Autodesk Inventor part; units mm, degrees
ref_plane "YZ Plane" through (0, 0, 0) normal (1, 0, 0) x (0, 1, 0)
ref_plane "XZ Plane" through (0, 0, 0) normal (0, 1, 0) x (-1, 0, 0)
ref_plane "XY Plane" through (0, 0, 0) normal (0, 0, 1) x (1, 0, 0)
sketch "Sketch1" plane through (0, 0, 0) normal (0, 0, 1) x (1, 0, 0)
  line L0 (0, 0) -> (190.5, 0)
  line L1 (190.5, 0) -> (190.5, 254)
  line L2 (190.5, 254) -> (0, 254)
  line L3 (0, 254) -> (0, 0)
  dimension "d0" = 190.5
  dimension "d1" = 254
extrude "Extrusion1" add sketch "Sketch1" against normal blind 25.4
sketch "Sketch2" plane through (0, 0, 0) normal (0, 0, 1) x (1, 0, 0)
  line L0 (0, 0) -> (0, 254)
  line L1 (0, 127) -> (190.5, 127)
  line L2 (190.5, 254) -> (190.5, 0)
  line L3 (54.1274, 112.395) -> (54.1274, 106.045)
  line L4 (95.25, 144.145) -> (117.3226, 144.145)
  line L5 (117.3226, 144.145) -> (73.1774, 144.145)
  line L6 (95.25, 109.855) -> (117.3226, 109.855)
  line L7 (117.3226, 109.855) -> (73.1774, 109.855)
  line L8 (73.1774, 144.145) -> (117.3226, 144.145)
  line L9 (117.3226, 144.145) -> (117.3226, 150.495)
  line L10 (117.3226, 150.495) -> (73.1774, 150.495)
  line L11 (73.1774, 150.495) -> (73.1774, 144.145)
  line L12 (73.1774, 109.855) -> (117.3226, 109.855)
  line L13 (117.3226, 109.855) -> (117.3226, 103.505)
  line L14 (117.3226, 103.505) -> (73.1774, 103.505)
  line L15 (73.1774, 103.505) -> (73.1774, 109.855)
  point P0 (54.1274, 141.605)
  dimension "d16" = 22.0726
  dimension "d17" = 44.1452
  dimension "d18" = 6.35
  dimension "d19" = 6.35
extrude "Extrusion2" add sketch "Sketch2" along normal blind 76.2
sketch "Sketch3" plane through (54.1274, 112.395, 0) normal (0, 1, 0) x (1, 0, 0)
  circle A0 centre (22.0726, -63.5) radius 6.35
  point P0 (-54.1274, 0)
  dimension "d10" = 12.7
extrude "Extrusion3" [suppressed]
sketch "Sketch4" plane through (0, 0, -25.4) normal (0, 0, -1) x (-1, 0, 0)
  line L0 (-190.5, 0) -> (-190.5, 254)
  line L1 (0, 0) -> (-190.5, 0)
  line L2 (-190.5, 0) -> (-190.5, 12.7)
  line L3 (-190.5, 12.7) -> (0, 12.7)
  line L4 (0, 12.7) -> (0, 0)
  dimension "d13" = 12.7
extrude "Extrusion4" add sketch "Sketch4" along normal blind 228.6
sketch "Sketch5" plane through (73.1774, 150.495, 0) normal (0, 1, 0) x (1, 0, 0)
  circle A0 centre (22.0726, -63.5) radius 6.35
  point P0 (-73.1774, 0)
  dimension "d20" = 12.7
extrude "Extrusion5" cut sketch "Sketch5" against normal blind 101.6
properties part number "LucasCharles Part3" material "ABS Plastic"
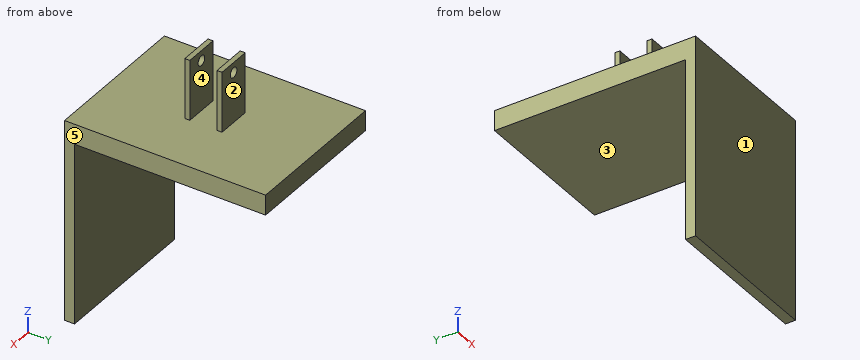
Design review of the part built by this model. Coordinates are the model's own, in mm. Face numbers are marked on the shaded views. A direction names the side the tool comes from. Round coordinates to 2 decimals unless told otherwise and drop trailing zeros. Write each loop counter-clockwise with the first axis right and the second up, starting at its lowest first coordinate (ties: lowest second). Pieces come first, ordered by that corner, then holes. Notation, with made-up numbers: (73.5, -25) - (85.5, -25) arc R38 cw to (85.5, 13) - close; hole circle Ø6 at (4.5, 61). An arc over 180 degrees is marked (long way). Use a Markdown table: item, result. Add a question column.
1. We need section B-B (z = 63.5). State the section outline as (x, y) points (3 decimals).
2. Wall thickness on probe 1 along X at (y, z) = (148, 63); probe 2 along Z at (x, y) = (95.25, 148); probe 3 along Y at (x, z) = (88, 32) (3 decimals): over which ranges is each line inside the solid? List them lowest first.
3. For the marked faces 1, 2, 3, 4 and 5, list the 3-axis set-ups (+Z, -Z, +X, -X, +Y, -Y) from which the entire face can be reached by the end or side of a thin tool; tool diameter is ignored.
4. We need section D-D (x = 33.5). State the section outline as (y, z) points, then the cut area to 3 significant figures.
5. We need section C-C (z = 6). State the section outline as (x, y) points (3 decimals), then the cut area to 3 significant figures.
6. We need section A-A (x = 95.25). State the section outline as (y, z) points (3 decimals).
7. Clearance check with flat-ended pins moving along their axes: pin 1 (7 mm diameter, centred on y = 106.5, z = 30.5, fed in from +X); pin 2 (13 mm diameter, centred on x = 93, z = 46, fed in from +Y) (3 decimals); pin 3 (4 mm diameter, centred on y = 104.5, z = 33, fed in from -X); pin 4 (11.5 mm diameter, centred on x = 95.25, z = 63.5, fed in from +Y). State where each tip first meets the part, or that it passes through.
Output:
| question | item | result |
|---|---|---|
| 1 | outline | (73.177, 103.505) - (88.9, 103.505) - (88.9, 109.855) - (73.177, 109.855) - close; (73.177, 144.145) - (88.9, 144.145) - (88.9, 150.495) - (73.177, 150.495) - close; (101.6, 103.505) - (117.323, 103.505) - (117.323, 109.855) - (101.6, 109.855) - close; (101.6, 144.145) - (117.323, 144.145) - (117.323, 150.495) - (101.6, 150.495) - close |
| 2 | probe 1 | x = 73.18 to 88.92, 101.58 to 117.32 |
| 2 | probe 2 | z = -25.4 to 57.15, 69.85 to 76.2 |
| 2 | probe 3 | y = 103.505 to 109.855, 144.145 to 150.495 |
| 3 | face 1 | +Z, -Z, +X, -X, -Y |
| 3 | face 2 | +Z, +X, -X, +Y |
| 3 | face 3 | -Z, +X, -X, +Y |
| 3 | face 4 | +Z, +X, -X |
| 3 | face 5 | +Z, -Z, +X, +Y, -Y |
| 4 | outline | (0, -254) - (12.7, -254) - (12.7, -25.4) - (254, -25.4) - (254, 0) - (0, 0) - close |
| 4 | area | 9,350 mm2 |
| 5 | outline | (73.177, 103.505) - (117.323, 103.505) - (117.323, 109.855) - (73.177, 109.855) - close; (73.177, 144.145) - (117.323, 144.145) - (117.323, 150.495) - (73.177, 150.495) - close |
| 5 | area | 561 mm2 |
| 6 | outline | (0, -254) - (12.7, -254) - (12.7, -25.4) - (254, -25.4) - (254, 0) - (150.495, 0) - (150.495, 57.15) - (144.145, 57.15) - (144.145, 0) - (109.855, 0) - (109.855, 57.15) - (103.505, 57.15) - (103.505, 0) - (0, 0) - close; (103.505, 69.85) - (109.855, 69.85) - (109.855, 76.2) - (103.505, 76.2) - close; (144.145, 69.85) - (150.495, 69.85) - (150.495, 76.2) - (144.145, 76.2) - close |
| 7 | pin 1 | stops at x = 117.32 |
| 7 | pin 2 | stops at y = 150.495 |
| 7 | pin 3 | stops at x = 73.18 |
| 7 | pin 4 | passes through |
